```python
from build123d import *

# Parameters (mm, degrees)
F0_W        = 40
F0_H        = 34
F0_R        = 2.05
F0_R_2      = 2.1
F1_DEPTH    = 5
F2_R        = 4.75
F2_R_2      = 2.1
F3_DEPTH    = 3
F4_W        = 24.05
F4_H        = 24.05
F4_W_2      = 20.2
F4_H_2      = 20.2
F5_DEPTH    = 30
F6_R        = 5
F7_R        = 4
F8_W        = 2
F8_H        = 4.975
F8_W_2      = 7.975
F8_H_2      = 2
F9_DEPTH    = 20
F10_SIZE2   = 19.2323419362
F10_SIZE    = 7
F10_2_SIZE2 = 19.2323419362
F10_2_SIZE  = 7
F11_SIZE2   = 7
F11_SIZE    = 19.2323419362
F12_SIZE2   = 4
F12_SIZE    = 10.9899096778
F13_SIZE2   = 10.9899096778
F13_SIZE    = 4
F13_2_SIZE2 = 10.9899096778
F13_2_SIZE  = 4


with BuildPart() as f1:
    # F0 (on Top) → F1 (new body)
    with BuildSketch(Plane.XY):
        Rectangle(F0_W, F0_H)
        with Locations((-15, -12)):
            Circle(F0_R, mode=Mode.SUBTRACT)
        with Locations((15, -12)):
            Circle(F0_R, mode=Mode.SUBTRACT)
        with Locations((-15, 12)):
            Circle(F0_R, mode=Mode.SUBTRACT)
        Circle(F0_R_2, mode=Mode.SUBTRACT)
        with Locations((15, 12)):
            Circle(F0_R, mode=Mode.SUBTRACT)
    extrude(amount=F1_DEPTH)

    # F2 (on face) → F3 (cut)
    with BuildSketch(Plane(origin=(0, 0, 0), x_dir=(1, 0, 0), z_dir=(0, 0, -1))):
        Circle(F2_R)
        Circle(F2_R_2, mode=Mode.SUBTRACT)
    extrude(amount=-F3_DEPTH, mode=Mode.SUBTRACT)

    # F4 (on face) → F5 (join)
    with BuildSketch(Plane.XY.offset(5)):
        Rectangle(F4_W, F4_H)
        Rectangle(F4_W_2, F4_H_2, mode=Mode.SUBTRACT)
    extrude(amount=F5_DEPTH)

    # F6
    f6_edges = [f1.edges().sort_by_distance(p)[0] for p in [
        (20, 17, 2.5),
        (20, -17, 2.5),
        (-20, -17, 2.5),
        (-20, 17, 2.5),
    ]]
    fillet(f6_edges, radius=F6_R)

    # F7
    f7_edges = [f1.edges().sort_by_distance(p)[0] for p in [
        (12.025, -12.025, 20),
        (12.025, 12.025, 20),
        (-12.025, -12.025, 20),
        (-12.025, 12.025, 20),
    ]]
    fillet(f7_edges, radius=F7_R)

    # F8 (on face) → F9 (join)
    with BuildSketch(Plane.XY.offset(5)):
        with Locations((-6, 14.5125)):
            Rectangle(F8_W, F8_H)
        with Locations((6, 14.5125)):
            Rectangle(F8_W, F8_H)
        with Locations((16.0125, 6)):
            Rectangle(F8_W_2, F8_H_2)
        with Locations((16.0125, -6)):
            Rectangle(F8_W_2, F8_H_2)
        with Locations((6, -14.5125)):
            Rectangle(F8_W, F8_H)
        with Locations((-6, -14.5125)):
            Rectangle(F8_W, F8_H)
        with Locations((-16.0125, -6)):
            Rectangle(F8_W_2, F8_H_2)
        with Locations((-16.0125, 6)):
            Rectangle(F8_W_2, F8_H_2)
    extrude(amount=F9_DEPTH)

    # F10
    f10_edges = [f1.edges().sort_by_distance(p)[0] for p in [
        (20, 6, 25),
    ]]
    f10_side = f1.faces().sort_by_distance((16.0125, 6, 25))[0]
    chamfer(f10_edges, length=F10_SIZE, length2=F10_SIZE2, reference=f10_side)

    # F10#2
    f10_2_edges = [f1.edges().sort_by_distance(p)[0] for p in [
        (20, -6, 25),
    ]]
    f10_2_side = f1.faces().sort_by_distance((16.0125, -6, 25))[0]
    chamfer(f10_2_edges, length=F10_2_SIZE, length2=F10_2_SIZE2, reference=f10_2_side)

    # F11
    f11_edges = [f1.edges().sort_by_distance(p)[0] for p in [
        (-20, 6, 25),
        (-20, -6, 25),
    ]]
    f11_side = f1.faces().sort_by_distance((-20, 0, 0.346554))[0]
    chamfer(f11_edges, length=F11_SIZE, length2=F11_SIZE2, reference=f11_side)

    # F12
    f12_edges = [f1.edges().sort_by_distance(p)[0] for p in [
        (6, -17, 25),
        (-6, -17, 25),
    ]]
    f12_side = f1.faces().sort_by_distance((0, -17, 0.390512))[0]
    chamfer(f12_edges, length=F12_SIZE, length2=F12_SIZE2, reference=f12_side)

    # F13
    f13_edges = [f1.edges().sort_by_distance(p)[0] for p in [
        (-6, 17, 25),
    ]]
    f13_side = f1.faces().sort_by_distance((-6, 14.5125, 25))[0]
    chamfer(f13_edges, length=F13_SIZE, length2=F13_SIZE2, reference=f13_side)

    # F13#2
    f13_2_edges = [f1.edges().sort_by_distance(p)[0] for p in [
        (6, 17, 25),
    ]]
    f13_2_side = f1.faces().sort_by_distance((6, 14.5125, 25))[0]
    chamfer(f13_2_edges, length=F13_2_SIZE, length2=F13_2_SIZE2, reference=f13_2_side)


solid = f1.part
```
Geometry check sheet. Reference: the model listing, model coordinates, mm. A direction names the side the tool comes from. Coordinates: 2 decimals unless noted, no trailing zeros. Order: outer loops, then holes, each group sorted by start corner. A loop starts at its lowest first (then second) coordinate and runs counter-clockwise, first axis right, second up. Notation, with made-up numbers: M 87,-10.5 L 113,-10.5 A29 cw 113,19.5 Z; hole C 48.5,50.25 d7. An arc over 180 degrees is marked long. One line per question, with ' | ' between items. Start each with the question number.
Item 1: Gauge pin test, flat ends, axial feed: pin 1 (1.5 mm diameter, centred on x = 0, y = 7, fed in from +Z); pin 2 (5 mm diameter, centred on y = 1.5, z = 19, fed in from -X) (3 decimals); pin 3 (1.5 mm diameter, centred on y = -15.5, z = 20, fed in from +X). Record the tip position at first contact, or that the pin passes through.
Item 2: Set-up check for faces 1 (the flat face through (6, 12.5, 25)), 2 (the flat face through (15, 7, 13)), 3 (the flat face through (15, -5, 13)), 4 (the flat face through (-7, -14, 13)): record each of +Z, -Z, +X, -X, +Y, -Y from which the full face is reachable in a straight line by a thin tool's end or side.
Item 3: Material ranges on L1, parallel to Y at x = 15, z = 1.85; L2, parallel to Y at x = 0, z = 1; L3, parallel to Y at x = 0, z = 4.35, recorded low to high. Write a range as [from, to].
Item 4: Draft check along X on faces 5 (the flat face through (15, -7, 13)), 6 (the flat face through (-10.1, 0, 20)), 7 (the flat face through (7, -14, 13)), 8 (the flat face through (-16.45, 5.99, 15.52)). Enter one of: pulls with the +X half, pulls with the -X half, needs draft (parallel to the pull), parting line crosses it, or undercut.
Item 5: Cross-section at A-A on x = 0. Enter the section's corners in (y, z) (3 decimals).
Item 6: Cross-section at C-C on y = 11. Enter the section's corners in (x, z), then the cut area to 3 significant figures.
Item 7: Cross-section at B-B on y = 0. Enter the section's corners in (x, z) (3 decimals), then the cut area to 3 significant figures.
Findings:
1) pin 1: stops at z = 5 | pin 2: stops at x = -12.025 | pin 3: stops at x = 7
2) face 1: +Z, +X, -X, +Y | face 2: +Z, +X, +Y | face 3: +Z, +X | face 4: +Z, -X, -Y
3) L1: y = [-17, -14.05], [-9.95, 9.95], [14.05, 17] | L2: y = [-17, -4.75], [4.75, 17] | L3: y = [-17, -2.1], [2.1, 17]
4) face 5: needs draft | face 6: undercut | face 7: pulls with the +X half | face 8: pulls with the -X half
5) outline: M -17,0 L -4.75,0 L -4.75,3 L -2.1,3 L -2.1,5 L -10.1,5 L -10.1,35 L -12.025,35 L -12.025,5 L -17,5 Z; M 2.1,3 L 4.75,3 L 4.75,0 L 17,0 L 17,5 L 12.025,5 L 12.025,35 L 10.1,35 L 10.1,5 L 2.1,5 Z
6) outline: M -20,0 L -16.79,0 L -16.79,5 L -20,5 Z; M -13.21,0 L 13.21,0 L 13.21,5 L 10.7,5 L 10.7,35 L -10.7,35 L -10.7,5 L -13.21,5 Z; M 16.79,0 L 20,0 L 20,5 L 16.79,5 Z | area: 806 mm²
7) outline: M -20,0 L -4.75,0 L -4.75,3 L -2.1,3 L -2.1,5 L -10.1,5 L -10.1,35 L -12.025,35 L -12.025,5 L -20,5 Z; M 2.1,3 L 4.75,3 L 4.75,0 L 20,0 L 20,5 L 12.025,5 L 12.025,35 L 10.1,35 L 10.1,5 L 2.1,5 Z | area: 279 mm²
